CAD build for the part. Positions are in the model's coordinates, mm. Face numbers are marked on the shaded views. A direction names the side the tool comes from. Give positions to 0.01 mm unless a question says otherwise; leave off trailing zeros. Loops run counter-clockwise (first coordinate to the right, second up) from the corner with the lowest first, then second, coordinate; pieces in that order, holes last.
```python
from build123d import *

# Parameters (mm, degrees)
SKETCH1_R               = 1.95
BOSS_EXTRUDE1_DEPTH     = 20
SKETCH2_R               = 3
CUT_EXTRUDE1_DEPTH      = 20
CUT_EXTRUDE1_DEPTH_BACK = 20


with BuildPart() as part:
    # Sketch1 → Boss-Extrude1 (new body)
    with BuildSketch(Plane.XY):
        with BuildLine():
            Line((3.143089642, 4.348706704), (4.348706704, 3.143089642))
            Line((4.348706704, 3.143089642), (2.930172249, 1.724555187))
            ThreePointArc((2.930172249, 1.724555187), (3.4, 0), (2.930172249, -1.724555187))
            Line((2.930172249, -1.724555187), (4.348706704, -3.143089642))
            Line((4.348706704, -3.143089642), (3.143089642, -4.348706704))
            Line((3.143089642, -4.348706704), (1.724555187, -2.930172249))
            ThreePointArc((1.724555187, -2.930172249), (0, -3.4), (-1.724555187, -2.930172249))
            Line((-1.724555187, -2.930172249), (-3.143089642, -4.348706704))
            Line((-3.143089642, -4.348706704), (-4.348706704, -3.143089642))
            Line((-4.348706704, -3.143089642), (-2.930172249, -1.724555187))
            ThreePointArc((-2.930172249, -1.724555187), (-3.4, 0), (-2.930172249, 1.724555187))
            Line((-2.930172249, 1.724555187), (-4.348706704, 3.143089642))
            Line((-4.348706704, 3.143089642), (-3.143089642, 4.348706704))
            Line((-3.143089642, 4.348706704), (-1.724555187, 2.930172249))
            ThreePointArc((-1.724555187, 2.930172249), (0, 3.4), (1.724555187, 2.930172249))
            Line((1.724555187, 2.930172249), (3.143089642, 4.348706704))
        make_face()
        Circle(SKETCH1_R, mode=Mode.SUBTRACT)
    extrude(amount=BOSS_EXTRUDE1_DEPTH)

    # Sketch2 → Cut-Extrude1 (cut, two sides)
    with BuildSketch(Plane(origin=(0, 0, 0), x_dir=(1, 0, 0), z_dir=(0, 1, 0))) as cut_extrude1_sk:
        with Locations((0, -11)):
            Circle(SKETCH2_R)
    extrude(amount=CUT_EXTRUDE1_DEPTH, mode=Mode.SUBTRACT)
    extrude(cut_extrude1_sk.sketch, amount=-CUT_EXTRUDE1_DEPTH_BACK, mode=Mode.SUBTRACT)


solid = part.part
```
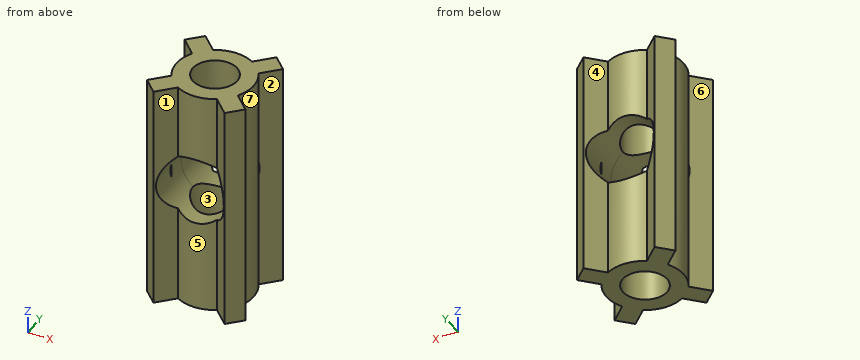
1. Tool access for the marked faces 1, 2, 3 and 4: list every direction of +Z, -Z, +X, -X, +Y, -Y with a clear straight run to the whole face (end or side of a thin tool).
Responses:
face 1: +Z, -Z, -Y
face 2: +Z, -Z, +X
face 3: +Z, -Z
face 4: +Z, -Z, +Y
2. Saw through at C-C, the plane x = -2.5. List the corners of the cut face in (y, z).
Responses:
outline: (-3.71, 0) - (3.71, 0) - (3.71, 9.34) - (-3.71, 9.34) - close; (-3.71, 12.66) - (3.71, 12.66) - (3.71, 20) - (-3.71, 20) - close
3. Probe line 1 along Y through (x, z) = (0, 3.25); line 2 along Z through (x, y) = (0, -3.25); line 3 along X through (y, z) = (-3, 11). List the from-to ranges inside material, lowest first.
Responses:
line 1: y = -3.4 to -1.95, 1.95 to 3.4
line 2: z = 0 to 8, 14 to 20
line 3: x = -4.21 to -3, 3 to 4.21
4. Saw through at A-A, the plane z = 3.5. List the corners of the cut face in (x, y), and give its area (3 significant figures).
Responses:
outline: (-4.35, -3.14) - (-3.14, -4.35) - (-1.72, -2.93) arc R3.4 ccw to (1.72, -2.93) - (3.14, -4.35) - (4.35, -3.14) - (2.93, -1.72) arc R3.4 ccw to (2.93, 1.72) - (4.35, 3.14) - (3.14, 4.35) - (1.72, 2.93) arc R3.4 ccw to (-1.72, 2.93) - (-3.14, 4.35) - (-4.35, 3.14) - (-2.93, 1.72) arc R3.4 ccw to (-2.93, -1.72) - close; hole circle Ø3.9 at (0, 0)
area: 37.6 mm2
5. Pull direction X, two halves, no side cores. Call the marked faces 5, 6 and 7: released by +X, released by -X, zero draft, split by the parting line, or undercut.
Responses:
face 5: undercut
face 6: released by -X
face 7: released by +X
6. Drop flat-ended pins along their axis: pin 1 (3 mm diameter, centred on x = 0, y = 0, fed in from +Z); pin 2 (1.5 mm diameter, centred on y = -2.5, z = 17, fed in from +X); pin 3 (3 mm diameter, centred on x = 2, z = 12, fed in from +Y); pin 4 (1.5 mm diameter, centred on x = 1, z = 4, fed in from +Y). Give the stop position or say it passes through.
Responses:
pin 1: passes through
pin 2: stops at x = 4.35
pin 3: stops at y = 4.35
pin 4: stops at y = 3.39
7. Saw through at D-D, the plane y = 0.5. List the corners of the cut face in (x, z), and give its area (3 significant figures).
Responses:
outline: (-3.36, 0) - (-1.88, 0) - (-1.88, 8.67) arc R3 cw to (-1.88, 13.33) - (-1.88, 20) - (-3.36, 20) - close; (1.88, 0) - (3.36, 0) - (3.36, 20) - (1.88, 20) - (1.88, 13.33) arc R3 cw to (1.88, 8.67) - close
area: 51.9 mm2
8. Saw through at B-B, the plane x = 0. List the corners of the cut face in (y, z).
Responses:
outline: (-3.4, 0) - (-1.95, 0) - (-1.95, 8) - (-3.4, 8) - close; (-3.4, 14) - (-1.95, 14) - (-1.95, 20) - (-3.4, 20) - close; (1.95, 0) - (3.4, 0) - (3.4, 8) - (1.95, 8) - close; (1.95, 14) - (3.4, 14) - (3.4, 20) - (1.95, 20) - close
